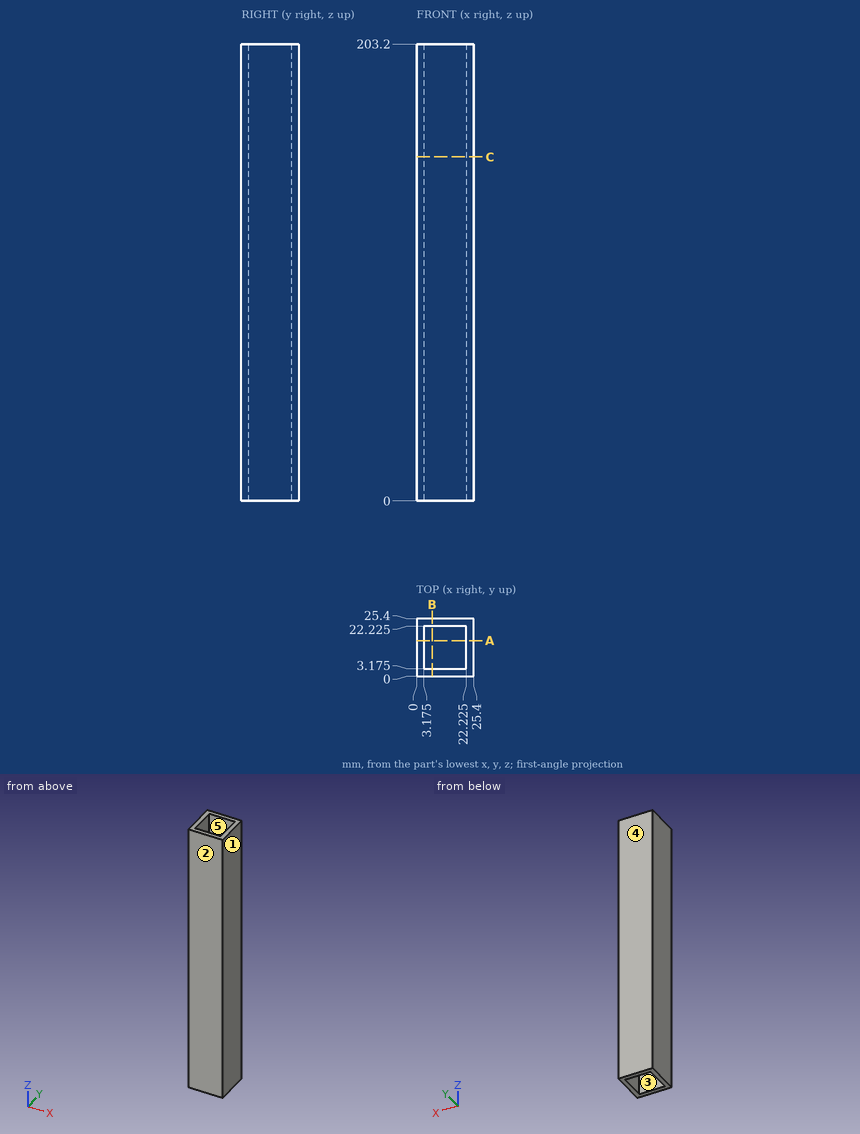
Print and shaded views of the part. All mm, measured from the part's lowest x, y and z. A direction names the side the tool comes from. Coordinates: 2 decimals unless noted, no trailing zeros. Order: outer loops, then holes, each group sorted by start corner. A loop starts at its lowest first (then second) coordinate and runs counter-clockwise, first axis right, second up. Notation, with made-up numbers: M 45.25,12.25 L 66.25,12.25 A18 ccw 66.25,21.25 Z; hole C 14,-30.5 d5. An arc over 180 degrees is marked long. One line per question, with ' | ' between items. Start each with the question number.
Q1. Probe L1, parallel to X at y = 16.5, z = 45 (3 decimals). List the from-to ranges inside material, lowest first. Write a range as from..to.
Q2. Two-plate mould, pull along X, no slides. Class the marked faces 1, 2 and 3: +X half, -X half, draft (parallel to the pull), parting line (faces both ways), or undercut.
Q3. Saw through at A-A (y = 15.75). List the corners of the cut face in (x, z) (3 decimals).
Q4. Saw through at C-C (z = 153). List the corners of the cut face in (x, y) (3 decimals).
Q5. 3-axis set-ups, long thin cutter, end or side, ignore diameter. For the marked faces 4 and 5: which of +Z, -Z, +X, -X, +Y, -Y reach the whole face in a straight line?
Check values:
1) L1: x = 0..3.175, 22.225..25.4
2) face 1: +X half | face 2: draft | face 3: undercut
3) outline: M 0,0 L 3.175,0 L 3.175,203.2 L 0,203.2 Z; M 22.225,0 L 25.4,0 L 25.4,203.2 L 22.225,203.2 Z
4) outline: M 0,0 L 25.4,0 L 25.4,25.4 L 0,25.4 Z; hole M 3.175,3.175 L 22.225,3.175 L 22.225,22.225 L 3.175,22.225 Z
5) face 4: +Z, -Z, +X, -X, +Y | face 5: +Z, -Z
